```python
from build123d import *

# Parameters (mm, degrees)
SKETCH1_W           = 63.5
SKETCH1_H           = 92.5
BOSS_EXTRUDE1_DEPTH = 1.5
BOSS_EXTRUDE2_START = 1.5
SKETCH1_2_W         = 63.5
SKETCH1_2_H         = 92.5
BOSS_EXTRUDE2_DEPTH = 1.75
SKETCH3_W           = 18.25
SKETCH3_H           = 12
CUT_EXTRUDE1_DEPTH  = 57.193304761
FILLET1_R           = 2.5
FILLET2_R           = 1.25
CUT_EXTRUDE2_DEPTH  = 57.193304761
SKETCH5_W           = 45.209659229
SKETCH5_H           = 5
BOSS_EXTRUDE3_DEPTH = 5.5
FILLET3_R           = 2.5


with BuildPart() as part:
    # Sketch1 → Boss-Extrude1 (new body)
    with BuildSketch(Plane.XY):
        Rectangle(SKETCH1_W, SKETCH1_H)
        with BuildLine():
            Line((-27, 43.9), (-13.75, 43.9))
            ThreePointArc((-13.75, 43.9), (-13.502512627, 44.002512627), (-13.4, 44.25))
            Line((-13.4, 44.25), (-13.4, 45))
            ThreePointArc((-13.4, 45), (-13.502512627, 45.247487373), (-13.75, 45.35))
            Line((-13.75, 45.35), (-28, 45.35))
            ThreePointArc((-28, 45.35), (-30.015254326, 44.515254326), (-30.85, 42.5))
            Line((-30.85, 42.5), (-30.85, 39.25))
            ThreePointArc((-30.85, 39.25), (-30.747487373, 39.002512627), (-30.5, 38.9))
            Line((-30.5, 38.9), (-29.75, 38.9))
            ThreePointArc((-29.75, 38.9), (-29.502512627, 39.002512627), (-29.4, 39.25))
            Line((-29.4, 39.25), (-29.4, 41.5))
            ThreePointArc((-29.4, 41.5), (-28.697056275, 43.197056275), (-27, 43.9))
        make_face(mode=Mode.SUBTRACT)
        with BuildLine():
            Line((30.85, -42.5), (30.85, 42.5))
            ThreePointArc((30.85, 42.5), (30.015254326, 44.515254326), (28, 45.35))
            Line((28, 45.35), (13.75, 45.35))
            ThreePointArc((13.75, 45.35), (13.502512627, 45.247487373), (13.4, 45))
            Line((13.4, 45), (13.4, 44.25))
            ThreePointArc((13.4, 44.25), (13.502512627, 44.002512627), (13.75, 43.9))
            Line((13.75, 43.9), (27, 43.9))
            ThreePointArc((27, 43.9), (28.697056275, 43.197056275), (29.4, 41.5))
            Line((29.4, 41.5), (29.4, -41.550510257))
            ThreePointArc((29.4, -41.550510257), (28.914537685, -42.997764711), (27.654545455, -43.859529583))
            ThreePointArc((27.654545455, -43.859529583), (27.470796588, -43.985203627), (27.4, -44.196261568))
            Line((27.4, -44.196261568), (27.4, -45))
            ThreePointArc((27.4, -45), (27.502512627, -45.247487373), (27.75, -45.35))
            Line((27.75, -45.35), (28, -45.35))
            ThreePointArc((28, -45.35), (30.015254326, -44.515254326), (30.85, -42.5))
        make_face(mode=Mode.SUBTRACT)
        with BuildLine():
            Line((-29.4, -41.550510257), (-29.4, -3.25))
            ThreePointArc((-29.4, -3.25), (-29.502512627, -3.002512627), (-29.75, -2.9))
            Line((-29.75, -2.9), (-30.5, -2.9))
            ThreePointArc((-30.5, -2.9), (-30.747487373, -3.002512627), (-30.85, -3.25))
            Line((-30.85, -3.25), (-30.85, -42.5))
            ThreePointArc((-30.85, -42.5), (-30.015254326, -44.515254326), (-28, -45.35))
            Line((-28, -45.35), (-27.75, -45.35))
            ThreePointArc((-27.75, -45.35), (-27.502512627, -45.247487373), (-27.4, -45))
            Line((-27.4, -45), (-27.4, -44.196261568))
            ThreePointArc((-27.4, -44.196261568), (-27.470796588, -43.985203627), (-27.654545455, -43.859529583))
            ThreePointArc((-27.654545455, -43.859529583), (-28.914537685, -42.997764711), (-29.4, -41.550510257))
        make_face(mode=Mode.SUBTRACT)
    extrude(amount=BOSS_EXTRUDE1_DEPTH)

    # Sketch1<2> → Boss-Extrude2 (add)
    with BuildSketch(Plane.XY.offset(BOSS_EXTRUDE2_START)):
        Rectangle(SKETCH1_2_W, SKETCH1_2_H)
    extrude(amount=BOSS_EXTRUDE2_DEPTH)

    # Sketch3 → Cut-Extrude1 (cut, through all)
    with BuildSketch(Plane.XY.offset(3.25)):
        with Locations((-19.125, -9.5)):
            Rectangle(SKETCH3_W, SKETCH3_H)
    extrude(amount=-CUT_EXTRUDE1_DEPTH, mode=Mode.SUBTRACT)

    # Fillet1
    fillet1_edges = [part.edges().sort_by_distance(p)[0] for p in [
        (-31.75, 46.25, 1.625),
        (31.75, 46.25, 1.625),
        (31.75, -46.25, 1.625),
        (-31.75, -46.25, 1.625),
    ]]
    fillet(fillet1_edges, radius=FILLET1_R)

    # Fillet2
    fillet2_edges = [part.edges().sort_by_distance(p)[0] for p in [
        (-28.25, -15.5, 1.625),
        (-28.25, -3.5, 1.625),
        (-10, -3.5, 1.625),
        (-10, -15.5, 1.625),
    ]]
    fillet(fillet2_edges, radius=FILLET2_R)

    # Sketch4 → Cut-Extrude2 (cut, through all)
    with BuildSketch(Plane.XY.offset(3.25)):
        with BuildLine():
            Line((-25, 37.5), (25, 37.5))
            ThreePointArc((25, 37.5), (26.25, 36.25), (25, 35))
            Line((25, 35), (-25, 35))
            ThreePointArc((-25, 35), (-26.25, 36.25), (-25, 37.5))
        make_face()
        with BuildLine():
            Line((-25, 32.5), (25, 32.5))
            ThreePointArc((25, 32.5), (26.25, 31.25), (25, 30))
            Line((25, 30), (-25, 30))
            ThreePointArc((-25, 30), (-26.25, 31.25), (-25, 32.5))
        make_face()
        with BuildLine():
            Line((-25, 27.5), (25, 27.5))
            ThreePointArc((25, 27.5), (26.25, 26.25), (25, 25))
            Line((25, 25), (-25, 25))
            ThreePointArc((-25, 25), (-26.25, 26.25), (-25, 27.5))
        make_face()
        with BuildLine():
            Line((-25, 22.5), (25, 22.5))
            ThreePointArc((25, 22.5), (26.25, 21.25), (25, 20))
            Line((25, 20), (-25, 20))
            ThreePointArc((-25, 20), (-26.25, 21.25), (-25, 22.5))
        make_face()
        with BuildLine():
            Line((-25, 17.5), (25, 17.5))
            ThreePointArc((25, 17.5), (26.25, 16.25), (25, 15))
            Line((25, 15), (-25, 15))
            ThreePointArc((-25, 15), (-26.25, 16.25), (-25, 17.5))
        make_face()
        with BuildLine():
            Line((-25, 12.5), (25, 12.5))
            ThreePointArc((25, 12.5), (26.25, 11.25), (25, 10))
            Line((25, 10), (-25, 10))
            ThreePointArc((-25, 10), (-26.25, 11.25), (-25, 12.5))
        make_face()
        with BuildLine():
            Line((-25, 7.5), (25, 7.5))
            ThreePointArc((25, 7.5), (26.25, 6.25), (25, 5))
            Line((25, 5), (-25, 5))
            ThreePointArc((-25, 5), (-26.25, 6.25), (-25, 7.5))
        make_face()
        with BuildLine():
            Line((-25, 2.5), (25, 2.5))
            ThreePointArc((25, 2.5), (26.25, 1.25), (25, 0))
            Line((25, 0), (-25, 0))
            ThreePointArc((-25, 0), (-26.25, 1.25), (-25, 2.5))
        make_face()
    extrude(amount=-CUT_EXTRUDE2_DEPTH, mode=Mode.SUBTRACT)

    # Sketch5 → Boss-Extrude3 (add)
    with BuildSketch(Plane(origin=(0, 0, 0), x_dir=(-1, 0, 0), z_dir=(0, 0, -1))):
        with Locations((1.138073126, -43.75)):
            Rectangle(SKETCH5_W, SKETCH5_H)
    extrude(amount=BOSS_EXTRUDE3_DEPTH)

    # Fillet3
    fillet3_edges = [part.edges().sort_by_distance(p)[0] for p in [
        (-23.74290274, -43.75, 0),
        (-1.138073126, -41.25, 0),
        (21.466756489, -43.75, 0),
    ]]
    fillet(fillet3_edges, radius=FILLET3_R)


solid = part.part
```
Geometry: final body of the model. Coordinates: model frame, mm. A direction names the side the tool comes from. Coordinates: 2 decimals unless noted, no trailing zeros. Order: outer loops, then holes, each group sorted by start corner. A loop starts at its lowest first (then second) coordinate and runs counter-clockwise, first axis right, second up. Notation, with made-up numbers: (-8, -33.5) - (34, -33.5) arc R31 ccw to (34, 3.5) - close; hole circle Ø8 at (6, 30.5). An arc over 180 degrees is marked (long way). Write each question's results on one line, items separated by ' | '.
(1) Section query C-C, the plane y = -30. Return the cut outline in (x, z), plus the area to 3 significant figures.
Values found:
outline: (-31.75, 0) - (-30.85, 0) - (-30.85, 1.5) - (-29.4, 1.5) - (-29.4, 0) - (29.4, 0) - (29.4, 1.5) - (30.85, 1.5) - (30.85, 0) - (31.75, 0) - (31.75, 3.25) - (-31.75, 3.25) - close | area: 202 mm²
(2) Section query A-A, the plane y = 31.25. Return the cut outline in (x, z).
Values found:
outline: (-31.75, 0) - (-26.25, 0) - (-26.25, 3.25) - (-31.75, 3.25) - close; (26.25, 0) - (29.4, 0) - (29.4, 1.5) - (30.85, 1.5) - (30.85, 0) - (31.75, 0) - (31.75, 3.25) - (26.25, 3.25) - close
(3) Section query B-B, the plane x = -20. Count the separate pieces of the cut face and the enclosed holes in it, plus the area to 3 significant figures.
Values found:
separate pieces: 10 | enclosed holes: 0 | area: 223 mm²
(4) Set-up query: faces 5 (the face through (-1, -41.25, -4)), 6 (the face through (-28.9, -43.02, 0.74)), 7 (the face through (26.25, 36.28, 1.65)). Return all of +Z, -Z, +X, -X, +Y, -Y with unobstructed straight access to the full face (end or side cutting, diameter ignored); none if empty.
Values found:
face 5: -Z, +X, -X, +Y | face 6: -Z | face 7: +Z, -Z
(5) Line query: line 1 (X direction, y = -11.5, z = 0.25); line 2 (X direction, y = 34.5, z = 1); line 3 (Z direction, x = 22, y = 14). Output: solid intervals per line, ascending. Write a range as [from, to].
Values found:
line 1: x = [-31.75, -30.85], [-29.4, -28.25], [-10, 29.4], [30.85, 31.75] | line 2: x = [-31.75, 29.4], [30.85, 31.75] | line 3: z = [0, 3.25]
(6) Mould query, pull axis Y, two halves, no side actions, for faces 1 (the face through (0, -46.25, -1)), 2 (the face through (-26.25, 16.22, 1.65)), 3 (the face through (0, 37.5, 2)), 4 (the face through (-23.743, -44, -4)). Classes: +Y half, -Y half, draft (parallel to the pull), parting line (faces both ways), or undercut.
Values found:
face 1: -Y half | face 2: undercut | face 3: undercut | face 4: draft
(7) First-contact query: pin 1 Ø12 at (x, y) = (2, -17.5) entering from -Z; pin 2 Ø1.5 at (y, z) = (-43.5, -4) entering from -X; pin 3 Ø2.5 at (x, z) = (-10, -3.5) entering from +Y. Flat tips, straight axial feed; report the tip coordinate or a pass-through.
Values found:
pin 1: stops at z = 0 | pin 2: stops at x = -23.74 | pin 3: stops at y = -41.24
